Build history of the part. All positions in model axes, mm. Round coordinates to 2 decimals unless told otherwise and drop trailing zeros. Write each loop counter-clockwise with the first axis right and the second up, starting at its lowest first coordinate (ties: lowest second). Pieces come first, ordered by that corner, then holes.
Item 1: Wall check: probe 1 along Y at (x, z) = (-1.3, 100); probe 2 along Y at (x, z) = (-1.4, 450); probe 3 along X at (y, z) = (5.25, 379). Give the ranges that are in metal, low to high.
Item 2: Band-saw the part on A-A, the plane z = 280.5. Write the cut outline in (x, y), then the cut area to 3 significant figures.
Item 3: Drop flat-ended pins along their axis: pin 1 Ø2.5 at (y, z) = (-1, -100) entering from +X; pin 2 Ø4.5 at (y, z) = (-1, 100) entering from +X; pin 3 Ø5 at (y, z) = (-1, 400) entering from +X. Give the stop position or say it passes through.
```python
from build123d import *

# Parameters (mm, degrees)
SKETCH1_W                      = 3
SKETCH1_H                      = 12
BOSS_EXTRUDE1_DEPTH            = 645
SKETCH2_R                      = 2
CUT_EXTRUDE1_DEPTH             = 10
CHAMFER1_SIZE                  = 2.5
CHAMFER2_SIZE                  = 1
LPATTERN1_COUNT                = 13
LPATTERN1_PITCH                = 50
CHAMFER1_OF_LPATTERN1_SIZE     = 2.5
LPATTERN1_COL_COUNT            = 13
LPATTERN1_COL_PITCH            = 50
CHAMFER1_OF_LPATTERN1_COL_SIZE = 2.5


with BuildPart() as part:
    # Sketch1 → Boss-Extrude1 (new, symmetric)
    with BuildSketch(Plane.XY):
        Rectangle(SKETCH1_W, SKETCH1_H)
    extrude(amount=BOSS_EXTRUDE1_DEPTH, both=True)

    # Sketch2 → Cut-Extrude1 (cut)
    with BuildSketch(Plane(origin=(1.5, 0, 0), x_dir=(0, 0, -1), z_dir=(1, 0, 0))):
        with Locations((0, -1)):
            Circle(SKETCH2_R)
    cut_extrude1 = extrude(amount=-CUT_EXTRUDE1_DEPTH, mode=Mode.SUBTRACT)

    # Chamfer1
    chamfer1_edges = [part.edges().sort_by_distance(p)[0] for p in [
        (1.5, -1, 2),
    ]]
    chamfer(chamfer1_edges, length=CHAMFER1_SIZE)

    # Chamfer2
    chamfer2_edges = [part.edges().sort_by_distance(p)[0] for p in [
        (-1.5, 6, 0),
        (1.5, 6, 0),
    ]]
    chamfer(chamfer2_edges, length=CHAMFER2_SIZE)

    # LPattern1: Cut-Extrude1 ×13
    with Locations(*[(0, 0, -i * LPATTERN1_PITCH) for i in range(1, LPATTERN1_COUNT)]):
        add(cut_extrude1, mode=Mode.SUBTRACT)

    # Chamfer1 of LPattern1
    chamfer1_of_lpattern1_edges = [part.edges().sort_by_distance(p)[0] for p in [
        (1.5, -1, -48),
        (1.5, -1, -98),
        (1.5, -1, -148),
        (1.5, -1, -198),
        (1.5, -1, -248),
        (1.5, -1, -298),
        (1.5, -1, -348),
        (1.5, -1, -398),
        (1.5, -1, -448),
        (1.5, -1, -498),
        (1.5, -1, -548),
        (1.5, -1, -598),
    ]]
    chamfer(chamfer1_of_lpattern1_edges, length=CHAMFER1_OF_LPATTERN1_SIZE)

    # LPattern1 col: Cut-Extrude1 ×13
    with Locations(*[(0, 0, i * LPATTERN1_COL_PITCH) for i in range(1, LPATTERN1_COL_COUNT)]):
        add(cut_extrude1, mode=Mode.SUBTRACT)

    # Chamfer1 of LPattern1 col
    chamfer1_of_lpattern1_col_edges = [part.edges().sort_by_distance(p)[0] for p in [
        (1.5, -1, 52),
        (1.5, -1, 102),
        (1.5, -1, 152),
        (1.5, -1, 202),
        (1.5, -1, 252),
        (1.5, -1, 302),
        (1.5, -1, 352),
        (1.5, -1, 402),
        (1.5, -1, 452),
        (1.5, -1, 502),
        (1.5, -1, 552),
        (1.5, -1, 602),
    ]]
    chamfer(chamfer1_of_lpattern1_col_edges, length=CHAMFER1_OF_LPATTERN1_COL_SIZE)


solid = part.part
```
Results:
1. probe 1: y = -6 to -3, 1 to 5.2
1. probe 2: y = -6 to -3, 1 to 5.1
1. probe 3: x = -1.25 to 1.25
2. outline: (-1.5, -6) - (1.5, -6) - (1.5, 5) - (0.5, 6) - (-0.5, 6) - (-1.5, 5) - close
2. area: 35.0 mm2
3. pin 1: passes through
3. pin 2: stops at x = -0.75
3. pin 3: stops at x = -0.5
